from build123d import *

# Parameters (mm, degrees)
SKETCH3_W           = 28.5
SKETCH3_H           = 51.8
BOSS_EXTRUDE4_DEPTH = 4
SKETCH7_W           = 4
SKETCH7_H           = 4
BOSS_EXTRUDE5_DEPTH = 5.5
SKETCH8_W           = 4
SKETCH8_H           = 4
BOSS_EXTRUDE6_DEPTH = 7
SKETCH10_R          = 1
CUT_EXTRUDE2_DEPTH  = 4
SKETCH11_W          = 8
SKETCH11_H          = 42
CUT_EXTRUDE3_DEPTH  = 36.185543907
FILLET2_R           = 1
FILLET3_R           = 2
SKETCH9_W           = 4
SKETCH9_H           = 8
SKETCH9_R           = 1.5
BOSS_EXTRUDE8_DEPTH = 2
FILLET4_R           = 2


with BuildPart() as part:
    # Sketch3 → Boss-Extrude4 (new body)
    with BuildSketch(Plane(origin=(0, 0, 0), x_dir=(-1, 0, 0), z_dir=(0, 0, 1))):
        Rectangle(SKETCH3_W, SKETCH3_H)
    extrude(amount=BOSS_EXTRUDE4_DEPTH)

    # Sketch7 → Boss-Extrude5 (add)
    with BuildSketch(Plane(origin=(0, 25.9, 0), x_dir=(1, 0, 0), z_dir=(0, 1, 0))):
        with Locations((-12.25, -2)):
            Rectangle(SKETCH7_W, SKETCH7_H)
        with Locations((12.25, -2)):
            Rectangle(SKETCH7_W, SKETCH7_H)
    boss_extrude5 = extrude(amount=BOSS_EXTRUDE5_DEPTH)

    # Mirror1: Boss-Extrude5 across plane
    add(boss_extrude5.mirror(Plane.ZX))

    # Sketch8 → Boss-Extrude6 (add)
    with BuildSketch(Plane.XY.offset(4)):
        with Locations((-12.25, 29.4)):
            Rectangle(SKETCH8_W, SKETCH8_H)
        with Locations((12.25, 29.4)):
            Rectangle(SKETCH8_W, SKETCH8_H)
        with Locations((12.25, -29.4)):
            Rectangle(SKETCH8_W, SKETCH8_H)
        with Locations((-12.25, -29.4)):
            Rectangle(SKETCH8_W, SKETCH8_H)
    extrude(amount=BOSS_EXTRUDE6_DEPTH)

    # Sketch10 → Cut-Extrude2 (cut)
    with BuildSketch(Plane.XY.offset(4)):
        with Locations((-11.78, 23.25)):
            Circle(SKETCH10_R)
        with Locations(Location((-11.78, -23.25, 0), (0, 0, 180))):
            Circle(SKETCH10_R)
        with Locations((11.78, -23.25)):
            Circle(SKETCH10_R)
        with Locations(Location((11.78, 23.25, 0), (0, 0, 180))):
            Circle(SKETCH10_R)
    extrude(amount=-CUT_EXTRUDE2_DEPTH, mode=Mode.SUBTRACT)

    # Sketch11 → Cut-Extrude3 (cut, through all)
    with BuildSketch(Plane.XY.offset(4)):
        with Locations((-10.25, 0)):
            Rectangle(SKETCH11_W, SKETCH11_H)
        with Locations((10.25, 0)):
            Rectangle(SKETCH11_W, SKETCH11_H)
    extrude(amount=-CUT_EXTRUDE3_DEPTH, mode=Mode.SUBTRACT)

    # Fillet2
    fillet2_edges = [part.edges().sort_by_distance(p)[0] for p in [
        (12.25, -27.4, 4),
        (-12.25, 27.4, 4),
    ]]
    fillet(fillet2_edges, radius=FILLET2_R)

    # Fillet3
    fillet3_edges = [part.edges().sort_by_distance(p)[0] for p in [
        (-10.25, -25.9, 2),
        (10.25, -25.9, 2),
        (-10.25, 25.9, 2),
        (10.25, 25.9, 2),
    ]]
    fillet(fillet3_edges, radius=FILLET3_R)

    # Sketch9 → Boss-Extrude8 (add)
    # profile 1 of 4: a face of its own
    with BuildSketch(Plane.XY.offset(11)):
        with Locations((-12.25, 31.4)):
            Rectangle(SKETCH9_W, SKETCH9_H)
        with Locations((-12.25, 33.4)):
            Circle(SKETCH9_R, mode=Mode.SUBTRACT)
    # profile 2 of 4: a face of its own
    with BuildSketch(Plane.XY.offset(11)):
        with Locations((12.25, 31.4)):
            Rectangle(SKETCH9_W, SKETCH9_H)
        with Locations(Location((12.25, 33.4, 0), (0, 0, 180))):
            Circle(SKETCH9_R, mode=Mode.SUBTRACT)
    # profile 3 of 4: a face of its own
    with BuildSketch(Plane.XY.offset(11)):
        with Locations((12.25, -31.4)):
            Rectangle(SKETCH9_W, SKETCH9_H)
        with Locations((12.25, -33.4)):
            Circle(SKETCH9_R, mode=Mode.SUBTRACT)
    # profile 4 of 4: a face of its own
    with BuildSketch(Plane.XY.offset(11)):
        with Locations((-12.25, -31.4)):
            Rectangle(SKETCH9_W, SKETCH9_H)
        with Locations(Location((-12.25, -33.4, 0), (0, 0, 180))):
            Circle(SKETCH9_R, mode=Mode.SUBTRACT)
    extrude(amount=BOSS_EXTRUDE8_DEPTH)

    # Fillet4
    fillet4_edges = [part.edges().sort_by_distance(p)[0] for p in [
        (-14.25, -21, 2),
        (-14.25, 21, 2),
        (-6.25, 21, 2),
        (-6.25, -21, 2),
        (6.25, 21, 2),
        (14.25, 21, 2),
        (14.25, -21, 2),
        (6.25, -21, 2),
        (-12.25, 31.4, 0),
        (-12.25, -27.4, 13),
        (12.25, 31.4, 0),
        (12.25, -27.4, 13),
        (12.25, 27.4, 13),
        (-12.25, 27.4, 13),
        (-12.25, -31.4, 0),
        (12.25, -31.4, 0),
    ]]
    fillet(fillet4_edges, radius=FILLET4_R)


solid = part.part
The model under review builds one solid part; all positions refer to its coordinate system, in mm. A direction names the side the tool comes from. Round coordinates to 2 decimals unless told otherwise and drop trailing zeros. Write each loop counter-clockwise with the first axis right and the second up, starting at its lowest first coordinate (ties: lowest second). Pieces come first, ordered by that corner, then holes. Notation, with made-up numbers: M -29,59 L 21,59 A17 ccw 21,77 Z; hole C -30,16.5 d10. An arc over 180 degrees is marked long. Answer as CSV lines item,"result". Start each with the question number.
Q1. The part is to be moulded in two halves that separate along X. For faces 1 (the face through (-9.9, -26.77, 2.98)), 2 (the face through (10.25, 30, 8)), 3 (the face through (-13.68, -21.6, 1.97)), 4 (the face through (-12, 35.4, 12)), say which applies: +X half, -X half, draft (parallel to the pull), parting line (faces both ways), or undercut.
Q2. Consider section C-C, the plane x = -0.5. Give the boundary of the cut face in (y, z).
Q3. Clearance check with flat-ended pins moving along their axes: P1, Ø3.5, axis at x = 12, z = 9, coming from the -Y side; P2, Ø2, axis at x = -11.5, z = 6, coming from the +Y side; P3, Ø1.5, axis at x = 6.5, y = 8.5, coming from the +Z side. State where each tip first meets the part, or that it passes through.
Q4. Consider section D-D, the plane y = 25. Give the boundary of the cut face in (x, z).
Q5. Tool access review of faces 5 (the face through (-11.925, -31.936, 11.986)), 6 (the face through (13, -35, 11)), 7 (the face through (14.25, -29, 5)), 8 (the face through (12.28, 28, 12.43)), 9 (the face through (6.82, -20.4, 1.97)): name each direction out of +Z, -Z, +X, -X, +Y, -Y from which nothing blocks a thin tool from reaching the whole face with its end or side.
Q6. Consider section A-A, the plane z = 7.75. Give the boundary of the cut face in (x, y).
Q7. Consider section B-B, the plane y = 33.4. Give the boundary of the cut face in (x, z), then the cut area to 3 significant figures.
Q8. Wall thickness on line 1 along Y through (x, z) = (11.78, 2.4); line 2 along Y through (x, z) = (12.5, 10.25); line 3 along X through (y, z) = (17, 3.25): over which ranges is each line inside the solid? List them lowest first.
Result set:
1,face 1,"undercut"
1,face 2,"undercut"
1,face 3,"-X half"
1,face 4,"draft"
2,outline,"M -25.9,0 L 25.9,0 L 25.9,4 L -25.9,4 Z"
3,P1,"stops at y = -31.4"
3,P2,"stops at y = 31.4"
3,P3,"stops at z = 4"
4,outline,"M -14.25,0 L 14.25,0 L 14.25,4 L -14.25,4 Z"
5,face 5,"+Z, -Z"
5,face 6,"-Z, +X, -X, -Y"
5,face 7,"+Z, -Z, +X, +Y, -Y"
5,face 8,"+Z, +X, -X"
5,face 9,"+Z, -Z, +X"
6,outline,"M -14.25,-31.4 L -10.25,-31.4 L -10.25,-27.9 A2 cw -10.19,-27.4 L -14.25,-27.4 Z; M -14.25,27.4 L -10.19,27.4 A2 cw -10.25,27.9 L -10.25,31.4 L -14.25,31.4 Z; M 10.19,-27.4 A2 cw 10.25,-27.9 L 10.25,-31.4 L 14.25,-31.4 L 14.25,-27.4 Z; M 10.19,27.4 L 14.25,27.4 L 14.25,31.4 L 10.25,31.4 L 10.25,27.9 A2 cw Z"
7,outline,"M -14.25,11 L -13.75,11 L -13.75,13 L -14.25,13 Z; M -10.75,11 L -10.25,11 L -10.25,13 L -10.75,13 Z; M 10.25,11 L 10.75,11 L 10.75,13 L 10.25,13 Z; M 13.75,11 L 14.25,11 L 14.25,13 L 13.75,13 Z"
7,area,"4.00 mm²"
8,line 1,"y = -31.4 to -24.25, -22.25 to -21, 21 to 22.25, 24.25 to 31.4"
8,line 2,"y = -31.4 to -27.4, 27.4 to 31.4"
8,line 3,"x = -6.25 to 6.25"
